For this review, use the dimensioned drawing (mm, ordinates from the lowest corner) and the shaded views. Give positions to 0.01 mm unless a question says otherwise; leave off trailing zeros. Order: outer loops, then holes, each group sorted by start corner. A loop starts at its lowest first (then second) coordinate and runs counter-clockwise, first axis right, second up. Notation, with made-up numbers: M 18,51.25 L 44,51.25 A18 cw 44,78.25 Z; hole C 54,72.5 d9. An arc over 180 degrees is marked long. Use CSV: the item, a comma, the result in double quotes. Start each with the question number.
(1) Wall thickness on L1, parallel to Y at x = 300, z = 55.5; L2, parallel to X at y = 82, z = 61.5; L3, parallel to X at y = 24, z = 52: over which ranges is each line inside the solid? List them lowest first. Write a range as from..to.
(2) Consider section A-A (x = 300). Write out the cut boundary in (y, z), and give its area (3 significant figures).
(3) Consider section D-D (x = 58.5). Write out the cut boundary in (y, z), and give its area (3 significant figures).
(4) Consider section C-C (x = 207). Write out the cut boundary in (y, z).
(5) Clearance check with flat-ended pins moving along their axes: P1, Ø8, axis at y = 66, z = 71, coming from the +X side; P2, Ø4, axis at x = 68, y = 23, coming from the +Z side; P3, Ø6, axis at x = 300, y = 49, coming from the -Z side. State where each tip first meets the part, or that it passes through.
(6) Consider section B-B (z = 53). Give the number of separate pieces and of enclosed holes in the cut face, and give its area (3 significant figures).
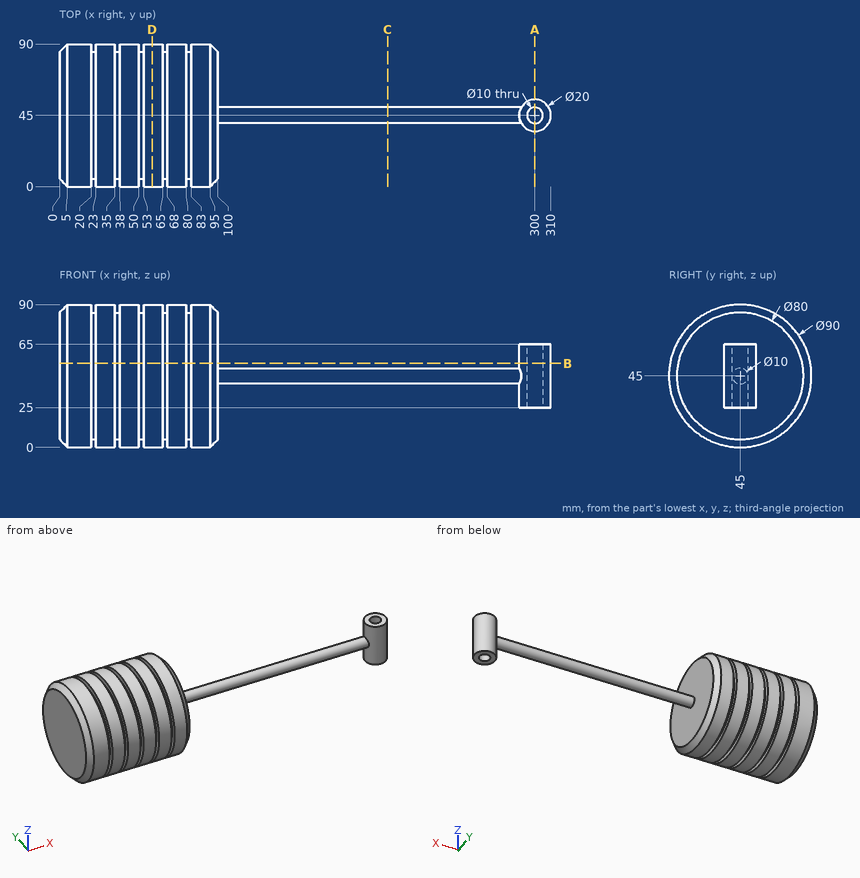
Check result:
1,L1,"y = 35..40, 50..55"
1,L2,"x = 0.51..20, 23..35, 38..50, 53..65, 68..80, 83..99.49"
1,L3,"x = 0..100"
2,outline,"M 35,25 L 40,25 L 40,65 L 35,65 Z; M 50,25 L 55,25 L 55,65 L 50,65 Z"
2,area,"400 mm^2"
3,outline,"C 45,45 d90"
3,area,"6,360 mm^2"
4,outline,"C 45,45 d10"
5,P1,"stops at x = 100"
5,P2,"stops at z = 85.31"
5,P3,"stops at z = 25"
6,separate pieces,"2"
6,enclosed holes,"1"
6,area,"8,890 mm^2"
